```python
from build123d import *

# Parameters (mm, degrees)
SKETCH_1_W                         = 600
SKETCH_1_H                         = 304
SM_BASE_FLANGE_1_DEPTH             = 1.5
SM_EDGE_FLANGE_1_STRIP_W           = 7.4732
SM_EDGE_FLANGE_1_STRIP_H           = 1.5
SM_EDGE_FLANGE_1_STRIP_CUT_DEPTH   = 600
SM_EDGE_FLANGE_1_STRIP_2_W         = 7.4732
SM_EDGE_FLANGE_1_STRIP_2_H         = 1.5
SM_EDGE_FLANGE_1_STRIP_CUT_2_DEPTH = 600
SM_EDGE_FLANGE_1_DEPTH             = 600
SM_EDGE_FLANGE_1_BEND_DEPTH        = 600
OTHER_START                        = -152
OTHER_1_DEPTH                      = 304
CUT_EXTRUDE_1_DEPTH                = 429.154177838
PATTERN_LINEAR_1_COUNT             = 3
PATTERN_LINEAR_1_PITCH             = 255


# Read off the part's stored shape, not the designer's step: 断开-边角1
# Sheet-metal steps are written as plain solids
with BuildPart() as part:
    # Sketch 1 → 基体-法兰1 (new body)
    with BuildSketch(Plane.XY):
        Rectangle(SKETCH_1_W, SKETCH_1_H)
    extrude(amount=-SM_BASE_FLANGE_1_DEPTH)

    # 边线-法兰1 strip (across the edge) → 边线-法兰1 strip cut (cut)
    with BuildSketch(Plane(origin=(300, -152, -1.5), x_dir=(0, 1, 0), z_dir=(-1, 0, 0))):
        with Locations((-1.5, -0.75)):
            Rectangle(SM_EDGE_FLANGE_1_STRIP_W, SM_EDGE_FLANGE_1_STRIP_H)
    extrude(amount=SM_EDGE_FLANGE_1_STRIP_CUT_DEPTH, mode=Mode.SUBTRACT)

    # 边线-法兰1 strip 2 (across the edge) → 边线-法兰1 strip cut 2 (cut)
    with BuildSketch(Plane(origin=(-300, 152, -1.5), x_dir=(0, -1, 0), z_dir=(1, 0, 0))):
        with Locations((-1.5, -0.75)):
            Rectangle(SM_EDGE_FLANGE_1_STRIP_2_W, SM_EDGE_FLANGE_1_STRIP_2_H)
    extrude(amount=SM_EDGE_FLANGE_1_STRIP_CUT_2_DEPTH, mode=Mode.SUBTRACT)

    # 边线-法兰1 section (across the edge) → 边线-法兰1 (add)
    with BuildSketch(Plane(origin=(300, -152, -1.5), x_dir=(0, 1, 0), z_dir=(-1, 0, 0))):
        with BuildLine():
            Line((0, 0.7366), (0, 28.5))
            Line((0, 28.5), (1.5, 28.5))
            Line((1.5, 28.5), (1.5, 0.7366))
            ThreePointArc((1.5, 0.7366), (1.715745145, 0.215745145), (2.2366, 0))
            Line((2.2366, 0), (2.2366, -1.5))
            ThreePointArc((2.2366, -1.5), (0.655084973, -0.844915027), (0, 0.7366))
        make_face()
    extrude(amount=SM_EDGE_FLANGE_1_DEPTH)

    # 边线-法兰1 section 2 (across the edge) → 边线-法兰1 bend (add)
    with BuildSketch(Plane(origin=(-300, 152, -1.5), x_dir=(0, -1, 0), z_dir=(1, 0, 0))):
        with BuildLine():
            Line((0, 0.7366), (0, 28.5))
            Line((0, 28.5), (1.5, 28.5))
            Line((1.5, 28.5), (1.5, 0.7366))
            ThreePointArc((1.5, 0.7366), (1.715745145, 0.215745145), (2.2366, 0))
            Line((2.2366, 0), (2.2366, -1.5))
            ThreePointArc((2.2366, -1.5), (0.655084973, -0.844915027), (0, 0.7366))
        make_face()
    extrude(amount=SM_EDGE_FLANGE_1_BEND_DEPTH)

    # Other 1 outline → Other 1 (cut)
    with BuildSketch(Plane(origin=(0, 0, 0), x_dir=(1, 0, 0), z_dir=(0, 1, 0)).offset(OTHER_START)):
        with BuildLine():
            Line((-300, 30), (-300, 27))
            ThreePointArc((-300, 27), (-299.121320344, 29.121320344), (-297, 30))
            Line((-297, 30), (-300, 30))
        make_face()
        with BuildLine():
            Line((300, 30), (297, 30))
            ThreePointArc((297, 30), (299.121320344, 29.121320344), (300, 27))
            Line((300, 27), (300, 30))
        make_face()
    extrude(amount=OTHER_1_DEPTH, mode=Mode.SUBTRACT)

    # 草图12 → 切除-拉伸1 (cut, symmetric)
    with BuildSketch(Plane.XZ.offset(152)):
        with BuildLine():
            Line((-254.5, -30), (-254.5, -20))
            ThreePointArc((-254.5, -20), (-250, -15.5), (-245.5, -20))
            Line((-245.5, -20), (-245.5, -30))
            ThreePointArc((-245.5, -30), (-250, -34.5), (-254.5, -30))
        make_face()
    cut_extrude_1 = extrude(amount=CUT_EXTRUDE_1_DEPTH, both=True, mode=Mode.SUBTRACT)

    # 阵列(线性)1: 切除-拉伸1 ×3
    with Locations(*[(i * PATTERN_LINEAR_1_PITCH, 0, 0) for i in range(1, PATTERN_LINEAR_1_COUNT)]):
        add(cut_extrude_1, mode=Mode.SUBTRACT)


solid = part.part
```
Part model, mm, in its own coordinate system. A direction names the side the tool comes from. Coordinates: 2 decimals unless noted, no trailing zeros. Write each loop counter-clockwise with the first axis right and the second up, starting at its lowest first coordinate (ties: lowest second). Pieces come first, ordered by that corner, then holes.
Item 1: Probe line 1 (Y direction, x = 178, z = -20.5); line 2 (Z direction, x = 104, y = -137). List the from-to ranges inside material, lowest first.
Item 2: Mould opens along Y. For faces 3 (the face through (-4, 150.5, -16)), 4 (the face through (-300, -1, -1)), 5 (the face through (4, -152, -13)) say: released by +Y, released by -Y, zero draft, split by the parting line, or undercut.
Item 3: Slice it at A-A (x = 236). Write the cut outline in (y, z), and give its area (3 significant figures).
Item 4: Slice it at B-B (y = 130). Write the cut outline in (x, z).
Item 5: Which spindle directions (+Z, -Z, +X, -X, +Y, -Y) get a long thin tool onto all of the face, cutting with end or side? Do faces 1 (the face through (-4, 2, -1.5)), 2 (the face through (-4, 2, 0)). Say none if no direction does.
Item 6: Pin check, flat tips, straight feed: pin 1 (10 mm diameter, centred on x = -133.5, y = 101.5, fed in from -Z); pin 2 (1 mm diameter, centred on x = -182.5, y = 94, fed in from +Z). Stop position of each tip, or through.
Results found:
1. line 1: y = -152 to -150.5, 150.5 to 152
1. line 2: z = -1.5 to 0
2. face 3: undercut
2. face 4: zero draft
2. face 5: released by -Y
3. outline: (-152, -30) - (-150.5, -30) - (-150.5, -2.24) arc R0.74 cw to (-149.76, -1.5) - (149.76, -1.5) arc R0.74 cw to (150.5, -2.24) - (150.5, -30) - (152, -30) - (152, -2.24) arc R2.24 ccw to (149.76, 0) - (-149.76, 0) arc R2.24 ccw to (-152, -2.24) - close
3. area: 540 mm2
4. outline: (-300, -1.5) - (300, -1.5) - (300, 0) - (-300, 0) - close
5. face 1: -Z, +X, -X
5. face 2: +Z, +X, -X, +Y, -Y
6. pin 1: stops at z = -1.5
6. pin 2: stops at z = 0
